Could you check a few things on this model? Use its own coordinates, in mm. Face numbers are marked on the shaded views. A direction names the side the tool comes from. Coordinates: 2 decimals unless noted, no trailing zeros. Order: outer loops, then holes, each group sorted by start corner. A loop starts at its lowest first (then second) coordinate and runs counter-clockwise, first axis right, second up. Notation, with made-up numbers: (34.25, 84) - (75.25, 84) arc R19 ccw to (75.25, 119) - close; hole circle Ø6 at (48, -11). An arc over 180 degrees is marked (long way). Answer as CSV lines item,"result". Start each with the question number.
1. I want a section at A-A, the plane x = 0. List the corners of the cut face in (y, z) for me.
2. I need wall thicknesses on probe 1 along Z at (x, y) = (-0.5, 0.5); probe 2 along Y at (x, z) = (-2, -6); probe 3 along Z at (x, y) = (12, -7.75). Which ranges of each line are inside material? Lowest first, please.
3. For pin 1 (4 mm diameter, centred on x = -9, y = 7, fed in from -Z); pin 2 (4 mm diameter, centred on y = -3.5, z = 18, fed in from -X); pin 3 (10 mm diameter, centred on x = 6.5, y = 2, fed in from +Z); pin 4 (10 mm diameter, centred on x = 2.5, y = 6.5, fed in from -Z), each with a flat end and sliding along its axis, tell me the tip position at first contact or that it passes through.
4. I want a section at C-C, the plane z = 0. List the corners of the cut face in (x, y) for me.
5. I want a section at B-B, the plane y = -4. List the corners of the cut face in (x, z) for me.
6. Thinking about a two-plate mould opening in X: for the marked faces 1, 2 and 3, which applies, released by +X, released by -X, zero draft, split by the parting line, or undercut?
7. For the marked faces 4 and 5, which set-ups out of +Z, -Z, +X, -X, +Y, -Y let a thin tool reach every point of the face, with its end or its side?
from build123d import *

# Parameters (mm, degrees)
SKETCH2_R           = 21.384776311
SKETCH2_W           = 26
SKETCH2_H           = 26
BOSS_EXTRUDE1_DEPTH = 10
SKETCH4_R           = 25
BOSS_EXTRUDE2_DEPTH = 2.5
FILLET1_R           = 2


with BuildPart() as part:
    # Sketch2 → Boss-Extrude1 (new, symmetric)
    with BuildSketch(Plane(origin=(0, 0, 0), x_dir=(1, 0, 0), z_dir=(0, 1, 0))):
        with Locations(Location((0, 0, 0), (0, 0, 270))):
            Circle(SKETCH2_R)
        Rectangle(SKETCH2_W, SKETCH2_H, mode=Mode.SUBTRACT)
    extrude(amount=BOSS_EXTRUDE1_DEPTH, both=True)

    # Sketch4 → Boss-Extrude2 (add)
    with BuildSketch(Plane(origin=(0, 10, 0), x_dir=(1, 0, 0), z_dir=(0, 1, 0))):
        with Locations(Location((0, 0, 0), (0, 0, 270))):
            Circle(SKETCH4_R)
    extrude(amount=BOSS_EXTRUDE2_DEPTH)

    # Fillet1
    fillet1_edges = [part.edges().sort_by_distance(p)[0] for p in [
        (0, 10, -21.384776311),
    ]]
    fillet(fillet1_edges, radius=FILLET1_R)


solid = part.part
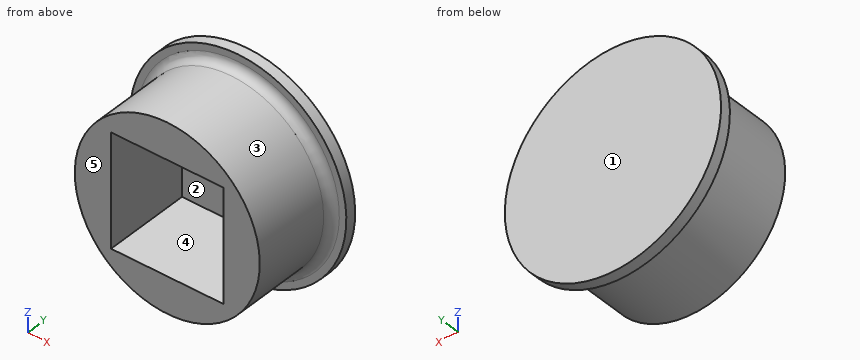
Solved:
1,outline,"(-10, -21.38) - (8, -21.38) arc R2 cw to (10, -23.38) - (10, -25) - (12.5, -25) - (12.5, 25) - (10, 25) - (10, 23.38) arc R2 cw to (8, 21.38) - (-10, 21.38) - (-10, 13) - (10, 13) - (10, -13) - (-10, -13) - close"
2,probe 1,"z = -21.38 to -13, 13 to 21.38"
2,probe 2,"y = 10 to 12.5"
2,probe 3,"z = -17.7 to -13, 13 to 17.7"
3,pin 1,"stops at z = -20.21"
3,pin 2,"stops at x = -14.19"
3,pin 3,"stops at z = 21.33"
3,pin 4,"stops at z = -25"
4,outline,"(-25, 10) - (-23.38, 10) arc R2 cw to (-21.38, 8) - (-21.38, -10) - (-13, -10) - (-13, 10) - (13, 10) - (13, -10) - (21.38, -10) - (21.38, 8) arc R2 cw to (23.38, 10) - (25, 10) - (25, 12.5) - (-25, 12.5) - close"
5,outline,"circle Ø42.77 at (0, 0); hole (-13, -13) - (13, -13) - (13, 13) - (-13, 13) - close"
6,face 1,"zero draft"
6,face 2,"undercut"
6,face 3,"split by the parting line"
7,face 4,"-Y"
7,face 5,"+Z, -Z, +X, -X, -Y"
